The drawing under review shows one solid part. Ordinate dimensions are in mm from its lowest x, y, z. A direction names the side the tool comes from. Coordinates: 2 decimals unless noted, no trailing zeros. Loops run counter-clockwise (first coordinate to the right, second up) from the corner with the lowest first, then second, coordinate; pieces in that order, holes last. Notation, with made-up numbers: (25.5, 10.5) - (47.5, 10.5) arc R4 cw to (47.5, 16.5) - close; hole circle Ø1 at (-34.5, 52). An arc over 180 degrees is marked (long way). Answer as a JSON object with one key per item and string values. Group by question number.
Item 1: Clearance check with a flat-ended pin moving along its axis: pin 1 (2 mm diameter, centred on x = 54.5, y = 63.5, fed in from +Z). State where the tip first meets the part, or that it passes through.
Item 2: We need section A-A (y = 47.5). Give the boundary of the cut face in (x, z) (1 decimal).
Item 3: We need section B-B (z = 22). Give the boundary of the cut face in (x, y) (1 decimal).
Item 4: To check wall thickness, follow line 1 (Z direction, x = 26, y = 23); line 2 (Y direction, x = 51.5, z = 3) (1 decimal); line 3 (Y direction, x = 40, z = 30.5) (1 decimal). State the ranges of each line that lie inside material, in increasing order.
Item 5: Tool access review of the marked faces 1 and 2: name each direction out of +Z, -Z, +X, -X, +Y, -Y from which nothing blocks a thin tool from reaching the whole face with its end or side.
Item 6: We need section D-D (y = 27). Give the boundary of the cut face in (x, z) (1 decimal).
Item 7: We need section C-C (x = 33.5). Give the boundary of the cut face in (y, z) (1 decimal), then the cut area to 4 significant figures.
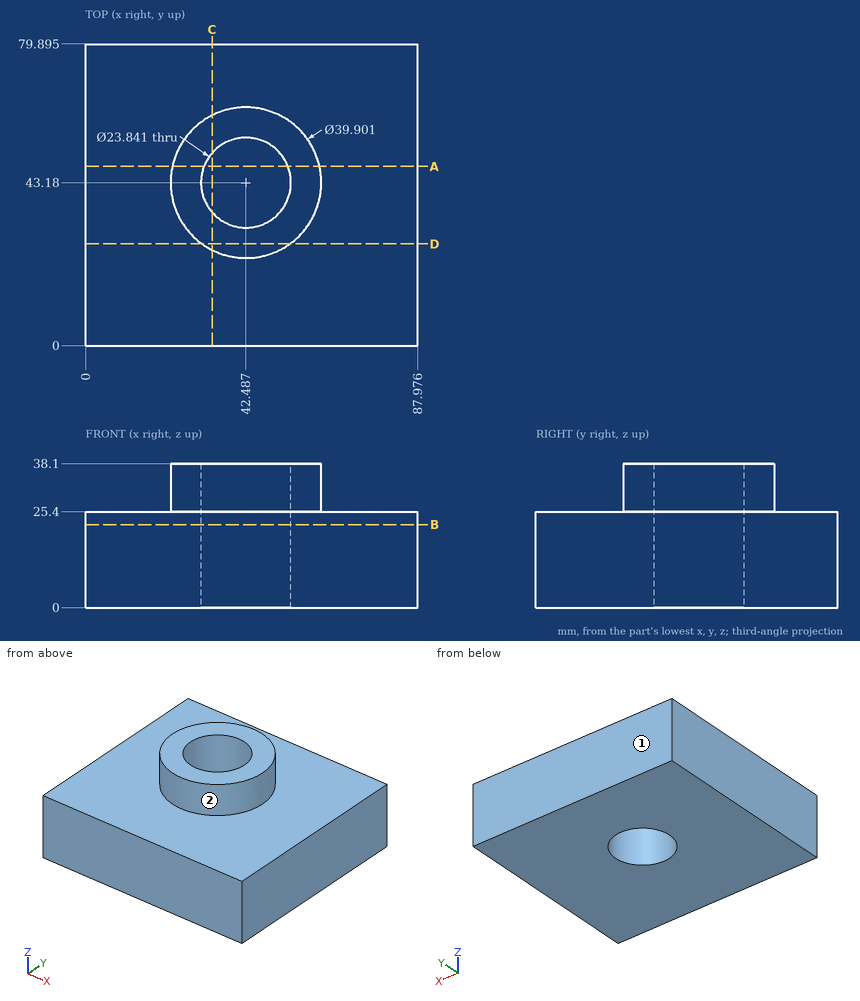
Check sheet entries:
{
 "1": {"pin 1": "stops at z = 25.4"},
 "2": {"outline": "(0, 0) - (31.4, 0) - (31.4, 38.1) - (23, 38.1) - (23, 25.4) - (0, 25.4) - close; (53.6, 0) - (88, 0) - (88, 25.4) - (62, 25.4) - (62, 38.1) - (53.6, 38.1) - close"},
 "3": {"outline": "(0, 0) - (88, 0) - (88, 79.9) - (0, 79.9) - close; hole circle Ø23.8 at (42.5, 43.2)"},
 "4": {"line 1": "z = 0 to 25.4", "line 2": "y = 0 to 35.4, 51 to 79.9", "line 3": "y = 23.4 to 31.5, 54.8 to 63"},
 "5": {"face 1": "+Z, -Z, +X, -X, +Y", "face 2": "+Z"},
 "6": {"outline": "(0, 0) - (88, 0) - (88, 25.4) - (54.2, 25.4) - (54.2, 38.1) - (30.8, 38.1) - (30.8, 25.4) - (0, 25.4) - close"},
 "7": {"outline": "(0, 0) - (35.3, 0) - (35.3, 38.1) - (25.4, 38.1) - (25.4, 25.4) - (0, 25.4) - close; (51, 0) - (79.9, 0) - (79.9, 25.4) - (61, 25.4) - (61, 38.1) - (51, 38.1) - close", "area": "1,885 mm2"}
}
